Part print with two shaded views. Sizes in mm from the minimum x, y, z corner. Coordinates: 2 decimals unless noted, no trailing zeros. Order: outer loops, then holes, each group sorted by start corner. A loop starts at its lowest first (then second) coordinate and runs counter-clockwise, first axis right, second up. Notation, with made-up numbers: (-14, 12.25) - (34, 12.25) arc R34 ccw to (34, 44.25) - close; hole circle Ø11 at (39.5, -1). An arc over 180 degrees is marked (long way). Return JSON: item names as keys, results as strings.
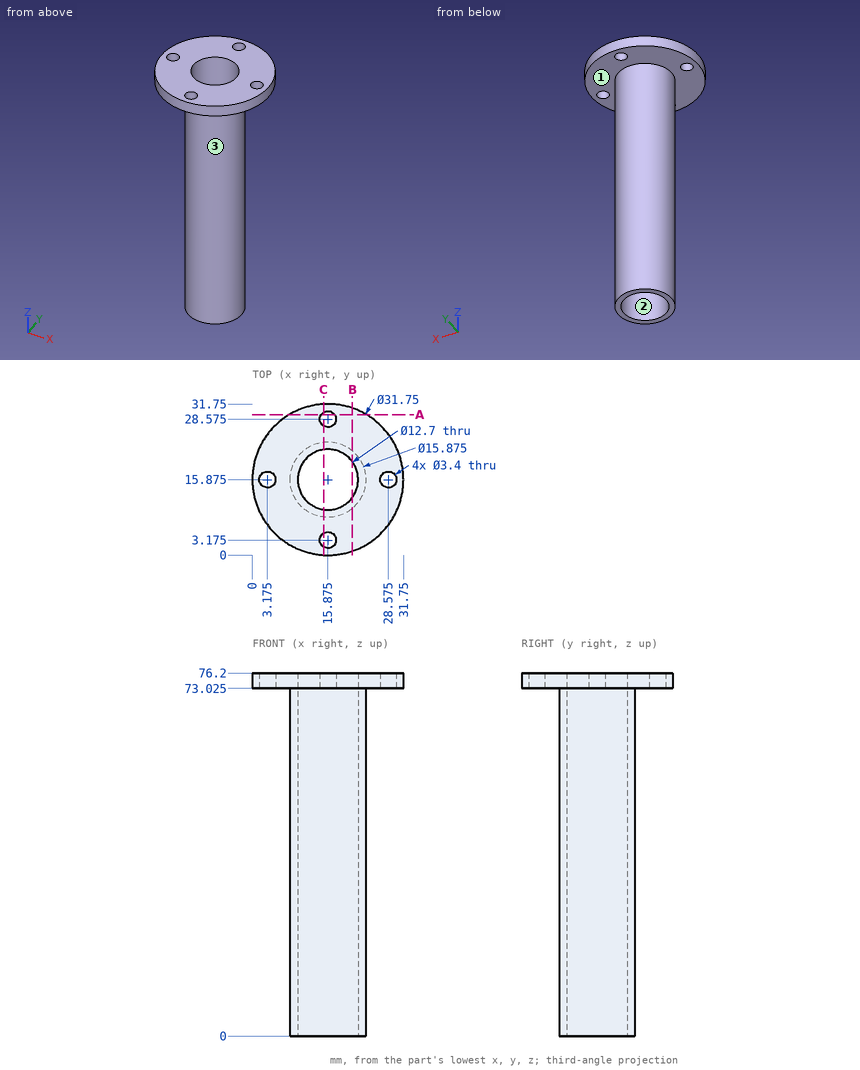
Item 1: Drop flat-ended pins along their axis: P1, Ø1, axis at x = 6, z = 20.5, coming from the -Y side; P2, Ø2, axis at y = 9.5, z = 36.5, coming from the -X side; P3, Ø4.5, axis at x = 15.875, y = 3.175, coming from the -Z side (3 decimals); P4, Ø2, axis at x = 23.5, z = 19, coming from the -Y side. Give the stop position or say it passes through.
Findings below:
{"P1": "passes through", "P2": "stops at x = 10.03", "P3": "stops at z = 73.025", "P4": "stops at y = 11.5"}
Item 2: Band-saw the part on C-C, the plane x = 15. List the corners of the cut face in (y, z) (3 decimals), then the cut area to 3 significant figures.
Findings below:
{"outline": "(0.024, 73.025) - (1.717, 73.025) - (1.717, 76.2) - (0.024, 76.2) - close; (4.633, 73.025) - (7.986, 73.025) - (7.986, 0) - (9.586, 0) - (9.586, 76.2) - (4.633, 76.2) - close; (22.164, 0) - (23.764, 0) - (23.764, 73.025) - (27.117, 73.025) - (27.117, 76.2) - (22.164, 76.2) - close; (30.033, 73.025) - (31.726, 73.025) - (31.726, 76.2) - (30.033, 76.2) - close", "area": "276 mm²"}
Item 3: Mould opens along X. For the marked faces 1, 2 and 3 say: released by +X, released by -X, zero draft, split by the parting line, or undercut.
Findings below:
{"face 1": "zero draft", "face 2": "undercut", "face 3": "split by the parting line"}
Item 4: Band-saw the part on A-A, the plane y = 29.5. List the corners of the cut face in (x, z) (3 decimals).
Findings below:
{"outline": "(7.728, 73.025) - (14.449, 73.025) - (14.449, 76.2) - (7.728, 76.2) - close; (17.301, 73.025) - (24.022, 73.025) - (24.022, 76.2) - (17.301, 76.2) - close"}
Item 5: Wall check: L1, parallel to X at y = 16, z = 12; L2, parallel to Y at x = 15.5, z = 27.5; L3, parallel to Z at x = 7, y = 26 (3 decimals). Give the ranges that are in metal, low to high. Write a range as [from, to].
Findings below:
{"L1": "x = [7.94, 9.53], [22.22, 23.81]", "L2": "y = [7.95, 9.54], [22.21, 23.8]", "L3": "z = [73.025, 76.2]"}
Item 6: Band-saw the part on B-B, the plane x = 21. List the corners of the cut face in (y, z) (3 decimals).
Findings below:
{"outline": "(0.85, 73.025) - (9.814, 73.025) - (9.814, 0) - (12.126, 0) - (12.126, 76.2) - (0.85, 76.2) - close; (19.624, 0) - (21.936, 0) - (21.936, 73.025) - (30.9, 73.025) - (30.9, 76.2) - (19.624, 76.2) - close"}
